Part model, mm, in its own coordinate system. A direction names the side the tool comes from. Coordinates: 2 decimals unless noted, no trailing zeros. Write each loop counter-clockwise with the first axis right and the second up, starting at its lowest first coordinate (ties: lowest second). Pieces come first, ordered by that corner, then holes. Notation, with made-up numbers: (44.5, 43.25) - (102.5, 43.25) arc R24 cw to (102.5, 74.25) - close; hole circle Ø2 at (-8.75, 9). An arc over 180 degrees is marked (long way). Write each question's results on one line, items separated by ' | '.
from build123d import *

# Parameters (mm, degrees)
SKETCH1_R           = 25
SKETCH1_R_2         = 1.8
SKETCH1_R_3         = 5.5
BOSS_EXTRUDE1_DEPTH = 7.5
SKETCH2_R           = 4
CUT_EXTRUDE1_DEPTH  = 6
BOSS_EXTRUDE2_START = -7.5
SKETCH3_R           = 33
SKETCH3_R_2         = 23
BOSS_EXTRUDE2_DEPTH = 47
SKETCH3_2_R         = 33
SKETCH3_2_R_2       = 23
BOSS_EXTRUDE3_DEPTH = 7.5
SKETCH7_W           = 40
SKETCH7_H           = 21.642183308
CUT_EXTRUDE3_DEPTH  = 25


with BuildPart() as part:
    # Sketch1 → Boss-Extrude1 (new body)
    with BuildSketch(Plane(origin=(0, 0, 0), x_dir=(1, 0, 0), z_dir=(0, 1, 0))):
        with Locations(Location((0, 0, 0), (0, 0, 270))):
            Circle(SKETCH1_R)
        with Locations(Location((-19, 0, 0), (0, 0, 270))):
            Circle(SKETCH1_R_2, mode=Mode.SUBTRACT)
        with Locations(Location((19, 0, 0), (0, 0, 90))):
            Circle(SKETCH1_R_2, mode=Mode.SUBTRACT)
        with Locations(Location((0, 0, 0), (0, 0, 270))):
            Circle(SKETCH1_R_3, mode=Mode.SUBTRACT)
    extrude(amount=BOSS_EXTRUDE1_DEPTH)

    # Sketch2 → Cut-Extrude1 (cut)
    with BuildSketch(Plane(origin=(0, 7.5, 0), x_dir=(1, 0, 0), z_dir=(0, 1, 0))):
        with Locations(Location((-19, 0, 0), (0, 0, 270))):
            Circle(SKETCH2_R)
        with Locations(Location((19, 0, 0), (0, 0, 270))):
            Circle(SKETCH2_R)
    extrude(amount=-CUT_EXTRUDE1_DEPTH, mode=Mode.SUBTRACT)

    # Sketch3 → Boss-Extrude2 (add)
    with BuildSketch(Plane.XZ.offset(BOSS_EXTRUDE2_START)):
        with Locations(Location((0, 0, 0), (0, 0, 90))):
            Circle(SKETCH3_R)
        with Locations(Location((0, 0, 0), (0, 0, 180.000077522))):
            Circle(SKETCH3_R_2, mode=Mode.SUBTRACT)
    extrude(amount=-BOSS_EXTRUDE2_DEPTH)

    # Sketch3<2> → Boss-Extrude3 (add)
    with BuildSketch(Plane.XZ):
        with Locations(Location((0, 0, 0), (0, 0, 270))):
            Circle(SKETCH3_2_R)
        with Locations(Location((0, 0, 0), (0, 0, 180.000077522))):
            Circle(SKETCH3_2_R_2, mode=Mode.SUBTRACT)
    extrude(amount=-BOSS_EXTRUDE3_DEPTH)

    # Sketch6 → Cut-Revolve7 (revolve, cut)
    with BuildSketch(Plane.XY, mode=Mode.PRIVATE) as cut_revolve7_sk:
        with BuildLine():
            Line((-33, 33.6), (-33, 54.5))
            Line((-33, 54.5), (-23, 54.5))
            Line((-23, 54.5), (-23, 33.6))
            add(Edge.make_bspline(
                [(-23, 33.6), (-23, 54.4), (-28, 54.4), (-33, 54.4), (-33, 33.6)],
                knots=[1.570796327, 1.570796327, 1.570796327, 3.141592654, 3.141592654, 4.71238898, 4.71238898, 4.71238898], degree=2, weights=[1, 0.707106781, 1, 0.707106781, 1]))
        make_face()
    revolve(cut_revolve7_sk.sketch.rotate(Axis((0, 54.5, 0), (0, -1, 0)), 90), axis=Axis((0, 54.5, 0), (0, -1, 0)), mode=Mode.SUBTRACT)

    # Sketch7 → Cut-Extrude3 (cut)
    with BuildSketch(Plane(origin=(0, 7.5, 0), x_dir=(1, 0, 0), z_dir=(0, 1, 0))):
        with Locations((0, 22.178908346)):
            Rectangle(SKETCH7_W, SKETCH7_H)
    extrude(amount=CUT_EXTRUDE3_DEPTH, mode=Mode.SUBTRACT)


solid = part.part
(1) 3-axis set-ups, long thin cutter, end or side, ignore diameter. For faces 3 (the flat face through (-20, 20, -19)), 4 (the cylindrical face through (-17.215, 0.74, -0.234)), 5 (the cylindrical face through (-15.034, 4.542, -0.521)): which of +Z, -Z, +X, -X, +Y, -Y reach the whole face in a straight line?
Return value:
face 3: -Z | face 4: +Y, -Y | face 5: +Y
(2) Flat gauge pins, fed straight in: P1, Ø12, axis at x = 14, z = -9, coming from the +Y side; P2, Ø6, axis at x = -11, y = 18, coming from the +Z side; P3, Ø6, axis at x = -19, z = 0, coming from the -Y side; P4, Ø3, axis at x = -9, y = 37.5, coming from the -Z side. Where does each tip first touch, or does it go through?
Return value:
P1: stops at y = 7.5 | P2: stops at z = 32.02 | P3: stops at y = 0 | P4: stops at z = -32.05
(3) Two-plate mould, pull along X, no slides. Class faces 1 (the flat face through (-7, 0, 0)), 2 (the flat face through (5, 7.5, -5)): released by +X, released by -X, zero draft, split by the parting line, or undercut.
Return value:
face 1: zero draft | face 2: undercut
(4) Wall check: line 1 (X direction, y = 0.95, z = 0); line 2 (X direction, y = 3, z = 0); line 3 (Y direction, x = 1, z = -7.5). Give the ranges that are in metal, low to high. Write a range as from..to.
Return value:
line 1: x = -33..-20.8, -17.2..-5.5, 5.5..17.2, 20.8..33 | line 2: x = -33..-23, -15..-5.5, 5.5..15, 23..33 | line 3: y = 0..7.5
(5) Saw through at B-B on x = -19. Count the separate pieces of the cut face and the enclosed holes in it, then the cut area to 3 significant figures.
Return value:
separate pieces: 3 | enclosed holes: 0 | area: 1,190 mm^2
(6) Saw through at A-A on y = 15.5. Write the cut outline in (x, z), then the cut area to 3 significant figures.
Return value:
outline: (-20, -26.25) - (-20, -11.36) arc R23 cw (long way) to (20, -11.36) - (20, -26.25) arc R33 ccw (long way) to start | area: 1,310 mm^2
